The listing builds one solid part. Answer for the finished solid, in the listing's coordinates (mm). A direction names the side the tool comes from. Coordinates: 2 decimals unless noted, no trailing zeros. Order: outer loops, then holes, each group sorted by start corner. A loop starts at its lowest first (then second) coordinate and runs counter-clockwise, first axis right, second up. Notation, with made-up numbers: (66.5, 1.25) -> (110.5, 1.25) arc R22 cw to (110.5, 32.25) -> close; hole circle Ø8 at (-8, 55.25). An arc over 180 degrees is marked (long way). Return JSON: item names as keys, results as strings.
from build123d import *

# Parameters (mm, degrees)
F2_R     = 12.7
F3_DEPTH = 76.2


with BuildPart() as f1:
    # F0 (on Top) → F1 (revolve)
    with BuildSketch(Plane.XY):
        Polygon((0, 38.927556), (-25.4, 38.927556), (-25.4, -37.272444), (50.8, -37.272444), (50.8, 38.927556), (25.4, 38.927556), (25.4, 0), (0, 0), align=None)
    revolve(axis=Axis((12.7, -62.672444, 0), (1, 0, 0)))

    # F2 (on face) → F3 (cut, through all)
    with BuildSketch(Plane.YZ.offset(50.8)):
        with BuildLine():
            ThreePointArc((-32.192444, 0), (-19.492444, -12.7), (-6.792444, 0))
            ThreePointArc((-6.792444, 0), (-19.492444, 12.7), (-32.192444, 0))
        make_face()
        with BuildLine():
            ThreePointArc((-61.752998, -30.463353), (-70.733254, -52.143609), (-49.052998, -43.163353))
            ThreePointArc((-49.052998, -43.163353), (-52.772742, -34.183097), (-61.752998, -30.463353))
        make_face()
        with Locations((-105.852444, 0)):
            Circle(F2_R)
        with BuildLine():
            ThreePointArc((-61.752998, 30.463353), (-52.772742, 34.183097), (-49.052998, 43.163353))
            ThreePointArc((-49.052998, 43.163353), (-70.733254, 52.143609), (-61.752998, 30.463353))
        make_face()
    extrude(amount=-F3_DEPTH, mode=Mode.SUBTRACT)


solid = f1.part
1. For faces 4 (the face through (37.922, -164.174, 4.467)), 5 (the face through (25.4, -109, -44)), determine the directions among +Z, -Z, +X, -X, +Y, -Y from which every point of the face is accessible in a straight line to the end or side of a thin tool.
Answer block:
{"face 4": "+X, -X", "face 5": "none"}
2. Determine the mould class of faces 1 (the face through (12.522, -2.894, 18.825)), 2 (the face through (13.23, -118.54, 0.56)), 3 (the face through (50.8, -84, -21)) for opening direction Y: pulls with the +Y half, pulls with the -Y half, needs draft (parallel to the pull), parting line crosses it, or undercut.
Answer block:
{"face 1": "parting line crosses it", "face 2": "undercut", "face 3": "needs draft"}
3. The part is cut by section C-C on z = -70. Give the vertices of the cut face in (x, y), and give its area (3 significant figures).
Answer block:
{"outline": "(-25.4, -136.31) -> (0, -136.31) -> (0, 10.97) -> (-25.4, 10.97) -> close; (25.4, -136.31) -> (50.8, -136.31) -> (50.8, 10.97) -> (25.4, 10.97) -> close", "area": "7,480 mm2"}
4. Consider line 1 (X direction, y = -40, z = 77); line 2 (Z direction, x = 21, y = -59.5); line 3 (Y direction, x = -16, z = -9). Determine where each line is inside the solid, lowest interval first. Write a range as from..to.
Answer block:
{"line 1": "x = -25.4..0, 25.4..50.8", "line 2": "z = -62.59..-55.66, -30.66..-25.2, 25.2..30.66, 55.66..62.59", "line 3": "y = -163.87..-114.81, -96.89..-86.42, -38.92..-28.45, -10.53..38.53"}
5. The part is cut by section A-A on z = 0. Give the vertices of the cut face in (x, y), and give its area (3 significant figures).
Answer block:
{"outline": "(-25.4, -164.27) -> (0, -164.27) -> (0, -125.34) -> (25.4, -125.34) -> (25.4, -164.27) -> (50.8, -164.27) -> (50.8, -118.55) -> (-25.4, -118.55) -> close; (-25.4, -93.15) -> (50.8, -93.15) -> (50.8, -88.07) -> (-25.4, -88.07) -> close; (-25.4, -37.27) -> (50.8, -37.27) -> (50.8, -32.19) -> (-25.4, -32.19) -> close; (-25.4, -6.79) -> (50.8, -6.79) -> (50.8, 38.93) -> (25.4, 38.93) -> (25.4, 0) -> (0, 0) -> (0, 38.93) -> (-25.4, 38.93) -> close", "area": "5,760 mm2"}
6. Each of these flat-tipped pins is pushed along its axis until it touches: pin 1 Ø3 at (x, z) = (36.5, -80) entering from -Y; pin 2 Ø10 at (x, z) = (-7.5, -50.5) entering from -Y; pin 3 Ø10 at (y, z) = (-43.5, -2) entering from +X; pin 4 Ø12 at (x, y) = (22.5, -127) entering from +Z. Where does it stop, or does it pass through?
Answer block:
{"pin 1": "stops at y = -127.17", "pin 2": "stops at y = -153.51", "pin 3": "passes through", "pin 4": "stops at z = 82.66"}
7. The part is cut by section D-D on y = -121. Give the vertices of the cut face in (x, z).
Answer block:
{"outline": "(-25.4, -83.19) -> (0, -83.19) -> (0, -22.93) -> (25.4, -22.93) -> (25.4, -83.19) -> (50.8, -83.19) -> (50.8, 83.19) -> (25.4, 83.19) -> (25.4, 22.93) -> (0, 22.93) -> (0, 83.19) -> (-25.4, 83.19) -> close"}
8. The part is cut by section B-B on x = -5. Give the vertices of the cut face in (y, z).
Answer block:
{"outline": "circle Ø203.2 at (-62.67, 0); hole circle Ø25.4 at (-105.85, 0); hole circle Ø50.8 at (-62.67, 0); hole circle Ø25.4 at (-61.75, -43.16); hole circle Ø25.4 at (-61.75, 43.16); hole circle Ø25.4 at (-19.49, 0)"}
